Source: CAD feature listing. Evaluate the final solid. Frame: model axes, mm. A direction names the side the tool comes from. Round coordinates to 2 decimals unless told otherwise and drop trailing zeros. Write each loop counter-clockwise with the first axis right and the second up, starting at its lowest first coordinate (ties: lowest second). Pieces come first, ordered by that corner, then holes. Notation, with made-up numbers: M -28.75,39 L 3.25,39 A21 ccw 3.25,69 Z; hole C 43.25,53.25 d10. An arc over 180 degrees is marked long. Use a Markdown table: item, result.
```python
from build123d import *

# Parameters (mm, degrees)
SKETCH1_W           = 25
SKETCH1_H           = 40
SKETCH1_R           = 1
BOSS_EXTRUDE1_DEPTH = 5
SKETCH2_W           = 6.2
SKETCH2_H           = 6.2
CUT_EXTRUDE1_DEPTH  = 2.5


with BuildPart() as part:
    # Sketch1 → Boss-Extrude1 (new body)
    with BuildSketch(Plane.XY):
        with Locations((-0.5, 8.252788104)):
            Rectangle(SKETCH1_W, SKETCH1_H)
        with Locations((-5, -4.247211896)):
            Circle(SKETCH1_R, mode=Mode.SUBTRACT)
        with Locations((4, -4.247211896)):
            Circle(SKETCH1_R, mode=Mode.SUBTRACT)
        with BuildLine():
            Line((-6.2, 23.993504103), (-6.2, 3.993504103))
            ThreePointArc((-6.2, 3.993504103), (-8, 2.193504103), (-9.8, 3.993504103))
            Line((-9.8, 3.993504103), (-9.8, 23.993504103))
            ThreePointArc((-9.8, 23.993504103), (-8, 25.793504103), (-6.2, 23.993504103))
        make_face(mode=Mode.SUBTRACT)
        with BuildLine():
            Line((6.2, 23.993504103), (6.2, 3.993504103))
            ThreePointArc((6.2, 3.993504103), (8, 2.193504103), (9.8, 3.993504103))
            Line((9.8, 3.993504103), (9.8, 23.993504103))
            ThreePointArc((9.8, 23.993504103), (8, 25.793504103), (6.2, 23.993504103))
        make_face(mode=Mode.SUBTRACT)
    extrude(amount=BOSS_EXTRUDE1_DEPTH)

    # Sketch2 → Cut-Extrude1 (cut)
    with BuildSketch(Plane(origin=(0, 0, 0), x_dir=(-1, 0, 0), z_dir=(0, 0, -1))):
        with Locations((-4, -4.247211896)):
            Rectangle(SKETCH2_W, SKETCH2_H)
        with Locations((5, -4.247211896)):
            Rectangle(SKETCH2_W, SKETCH2_H)
    extrude(amount=-CUT_EXTRUDE1_DEPTH, mode=Mode.SUBTRACT)


solid = part.part
```
Q1. Section A-A on y = 20.5. Return loops of the section in (x, z), plus the area to 3 significant figures.
Results are:
| item | result |
|---|---|
| outline | M -13,0 L -9.8,0 L -9.8,5 L -13,5 Z; M -6.2,0 L 6.2,0 L 6.2,5 L -6.2,5 Z; M 9.8,0 L 12,0 L 12,5 L 9.8,5 Z |
| area | 89.0 mm^2 |
Q2. Reachability of faces 4 (the flat face through (12, 8, 2)), 5 (the flat face through (-5, -1.147, 1)), 6 (the flat face through (9.8, 14, 2)) from +Z, -Z, +X, -X, +Y, -Y: full face, straight path, thin tool, end or side. Return the list, or none.
Results are:
| item | result |
|---|---|
| face 4 | +Z, -Z, +X, +Y, -Y |
| face 5 | -Z |
| face 6 | +Z, -Z |
Q3. Line query: L1, parallel to X at y = 17, z = 4.85; L2, parallel to X at y = -7, z = 1.7; L3, parallel to Y at x = 3.5, z = 1.8. Output: solid intervals per line, ascending.
Results are:
| item | result |
|---|---|
| L1 | -13 to -9.8, -6.2 to 6.2, 9.8 to 12 |
| L2 | -13 to -8.1, -1.9 to 0.9, 7.1 to 12 |
| L3 | -11.75 to -7.35, -1.15 to 28.25 |
Q4. Section B-B on x = -5. Return loops of the section in (y, z), plus the area to 4 significant figures.
Results are:
| item | result |
|---|---|
| outline | M -11.75,0 L -7.35,0 L -7.35,2.5 L -5.25,2.5 L -5.25,5 L -11.75,5 Z; M -3.25,2.5 L -1.15,2.5 L -1.15,0 L 28.25,0 L 28.25,5 L -3.25,5 Z |
| area | 179.5 mm^2 |
Q5. Section C-C on z = 0.6. Return loops of the section in (x, y), plus the area to 3 significant figures.
Results are:
| item | result |
|---|---|
| outline | M -13,-11.75 L 12,-11.75 L 12,28.25 L -13,28.25 Z; hole M -9.8,3.99 A1.8 ccw -6.2,3.99 L -6.2,23.99 A1.8 ccw -9.8,23.99 Z; hole M -8.1,-7.35 L -1.9,-7.35 L -1.9,-1.15 L -8.1,-1.15 Z; hole M 0.9,-7.35 L 7.1,-7.35 L 7.1,-1.15 L 0.9,-1.15 Z; hole M 6.2,3.99 A1.8 ccw 9.8,3.99 L 9.8,23.99 A1.8 ccw 6.2,23.99 Z |
| area | 759 mm^2 |
Q6. First-contact query: pin 1 Ø1.8 at (x, y) = (-5, -4.25) entering from -Z. Flat tip, straight axial feed; report the tip coordinate or a pass-through.
Results are:
| item | result |
|---|---|
| pin 1 | through |
Q7. Mould query, pull axis Y, two halves, no side actions, for faces 1 (the flat face through (-1, 28.253, 2)), 2 (the flat face through (-1, 9, 0)), 3 (the cylindrical face through (-5.79, -4.86, 3.73)). Classes: +Y half, -Y half, draft (parallel to the pull), parting line (faces both ways), or undercut.
Results are:
| item | result |
|---|---|
| face 1 | +Y half |
| face 2 | draft |
| face 3 | undercut |
Q8. Section D-D on x = 8. Return loops of the section in (y, z), plus the area to 3 significant figures.
Results are:
| item | result |
|---|---|
| outline | M -11.75,0 L 2.19,0 L 2.19,5 L -11.75,5 Z; M 25.79,0 L 28.25,0 L 28.25,5 L 25.79,5 Z |
| area | 82.0 mm^2 |
